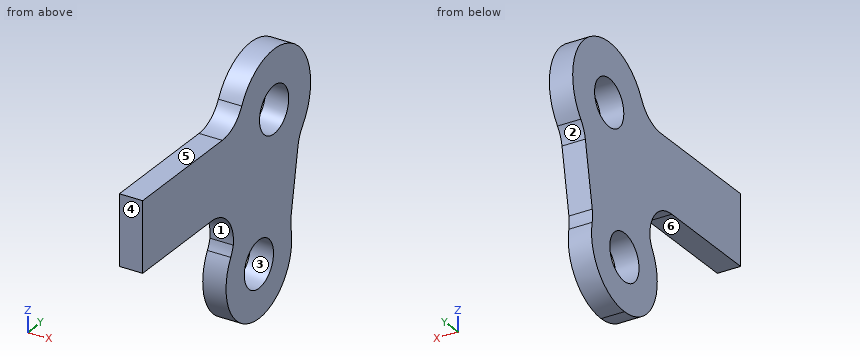
```python
from build123d import *

# Parameters (mm, degrees)
EXTRUDE_1_DEPTH          = 2
CUT_EXTRUDE_3_DEPTH      = 25.377594344
CUT_EXTRUDE_3_DEPTH_BACK = 25.377594344
SKETCH_1_3_R             = 2
FILLET_1_R               = 3


with BuildPart() as part:
    # 草图1 → 凸台-拉伸1 (new body)
    with BuildSketch(Plane(origin=(0, 0, 0), x_dir=(0, 0, -1), z_dir=(1, 0, 0))):
        with BuildLine():
            Line((0.694592711, 3.939231012), (-0.694592711, -3.939231012))
            Line((-0.694592711, -3.939231012), (3.079360166, -3.939231012))
            ThreePointArc((3.079360166, -3.939231012), (4.494263056, -2.191255253), (5, 0))
            ThreePointArc((5, 0), (4.650004293, 1.837786733), (3.64901597, 3.418286479))
            Line((3.64901597, 3.418286479), (0.694592711, 3.939231012))
        make_face()
        with BuildLine():
            Line((2.259830548, -4.460175545), (-0.694592711, -3.939231012))
            Line((-0.694592711, -3.939231012), (-0.694592711, -4.951519056))
            ThreePointArc((-0.694592711, -4.951519056), (0.820272506, -4.932256382), (2.259830548, -4.460175545))
        make_face()
        with BuildLine():
            Line((3.079360166, -3.939231012), (-0.694592711, -3.939231012))
            Line((-0.694592711, -3.939231012), (2.259830548, -4.460175545))
            ThreePointArc((2.259830548, -4.460175545), (2.68227239, -4.219646292), (3.079360166, -3.939231012))
        make_face()
        with BuildLine():
            Line((-0.694592711, -4.951519056), (-0.694592711, -3.939231012))
            Line((-0.694592711, -3.939231012), (0.694592711, 3.939231012))
            Line((0.694592711, 3.939231012), (3.64901597, 3.418286479))
            ThreePointArc((3.64901597, 3.418286479), (-4.437968609, 2.303135825), (-0.694592711, -4.951519056))
        make_face()
        with BuildLine():
            ThreePointArc((5, 0), (4.494263056, -2.191255253), (3.079360166, -3.939231012))
            Line((3.079360166, -3.939231012), (5.305407289, -3.939231012))
            Line((5.305407289, -3.939231012), (5.305407289, -4.997192896))
            Line((5.305407289, -4.997192896), (9.092867132, -5.665024255))
            ThreePointArc((9.092867132, -5.665024255), (7.386058148, -1.302361333), (10.482052554, 2.213437769))
            Line((10.482052554, 2.213437769), (3.64901597, 3.418286479))
            ThreePointArc((3.64901597, 3.418286479), (4.650004293, 1.837786733), (5, 0))
        make_face()
        with BuildLine():
            Line((5.305407289, -3.939231012), (3.079360166, -3.939231012))
            ThreePointArc((3.079360166, -3.939231012), (2.68227239, -4.219646292), (2.259830548, -4.460175545))
            Line((2.259830548, -4.460175545), (5.305407289, -4.997192896))
            Line((5.305407289, -4.997192896), (5.305407289, -3.939231012))
        make_face()
        with BuildLine():
            ThreePointArc((2.259830548, -4.460175545), (0.820272506, -4.932256382), (-0.694592711, -4.951519056))
            Line((-0.694592711, -4.951519056), (-0.694592711, -18))
            Line((-0.694592711, -18), (5.305407289, -18))
            Line((5.305407289, -18), (5.305407289, -4.997192896))
            Line((5.305407289, -4.997192896), (2.259830548, -4.460175545))
        make_face()
        with BuildLine():
            ThreePointArc((16.317693036, -2.083778132), (14.485990042, 1.539782422), (10.482052554, 2.213437769))
            Line((10.482052554, 2.213437769), (12.512285747, 1.85545288))
            Line((12.512285747, 1.85545288), (11.123100325, -6.023009144))
            Line((11.123100325, -6.023009144), (9.092867132, -5.665024255))
            ThreePointArc((9.092867132, -5.665024255), (13.816227929, -6.115633571), (16.317693036, -2.083778132))
        make_face()
        with BuildLine():
            Line((12.512285747, 1.85545288), (10.482052554, 2.213437769))
            ThreePointArc((10.482052554, 2.213437769), (7.386058148, -1.302361333), (9.092867132, -5.665024255))
            Line((9.092867132, -5.665024255), (11.123100325, -6.023009144))
            Line((11.123100325, -6.023009144), (12.512285747, 1.85545288))
        make_face()
    extrude(amount=EXTRUDE_1_DEPTH)

    # 草图1<3> → 切除-拉伸3 (cut, two sides: drawn at the far end of the back side and taken through both)
    with BuildSketch(Plane(origin=(0, 0, 0), x_dir=(0, 0, -1), z_dir=(1, 0, 0)).offset(-CUT_EXTRUDE_3_DEPTH_BACK)):
        Circle(SKETCH_1_3_R)
        with Locations((11.817693036, -2.083778132)):
            Circle(SKETCH_1_3_R)
    extrude(amount=CUT_EXTRUDE_3_DEPTH + CUT_EXTRUDE_3_DEPTH_BACK, mode=Mode.SUBTRACT)

    # 圆角1
    # the kernel refuses this fillet: 3 mm, written as the material it adds along each edge
    with BuildSketch(Plane(origin=(0, -4.951519056, 0.694592711), x_dir=(0, -1, 0), z_dir=(1, 0, 0))) as fillet_1_piece_1:
        with BuildLine():
            CenterArc((2.144253255, -3), FILLET_1_R, 90, 62.495124604)
            ThreePointArc((-0.516661362, -1.614527733), (-0.189409011, -0.829319334), (0, 0))
            Line((0, 0), (2.144253255, 0))
        make_face()
    extrude(amount=2)
    with BuildSketch(Plane(origin=(0, 3.418286479, -3.64901597), x_dir=(0, -0.17364817766699442, -0.9848077530121968), z_dir=(1, 0, 0))) as fillet_1_piece_2:
        with BuildLine():
            CenterArc((0.872983346, 3), FILLET_1_R, 241.044975628, 28.955024372)
            ThreePointArc((-0.579385409, 0.375), (-0.283214788, 0.19750856), (0, 0))
            Line((0, 0), (0.872983346, 0))
        make_face()
    extrude(amount=2)
    with BuildSketch(Plane(origin=(0, -4.997192896, -5.305407289), x_dir=(0, -0.17364817766692767, -0.9848077530122085), z_dir=(1, 0, 0))) as fillet_1_piece_3:
        with BuildLine():
            CenterArc((FILLET_1_R * 1.19175359259, -FILLET_1_R), FILLET_1_R, 90, 100)
            Line((FILLET_1_R * 0.206945839582, -FILLET_1_R * 1.17364817767), (0, 0))
            Line((0, 0), (FILLET_1_R * 1.19175359259, 0))
        make_face()
    extrude(amount=2)
    with BuildSketch(Plane(origin=(0, -5.665024255, -9.092867132), x_dir=(0, 0.17364817766698767, 0.9848077530121979), z_dir=(1, 0, 0))) as fillet_1_piece_4:
        with BuildLine():
            CenterArc((0.631029591, 3), FILLET_1_R, 248.960530219, 21.039469781)
            ThreePointArc((-0.446003371, 0.2), (-0.220284161, 0.106060125), (0, 0))
            Line((0, 0), (0.631029591, 0))
        make_face()
    extrude(amount=2)
    with BuildSketch(Plane(origin=(0, 2.213437769, -10.482052554), x_dir=(0, 0.2445079523565027, -0.9696472870247357), z_dir=(1, 0, 0))) as fillet_1_piece_5:
        with BuildLine():
            CenterArc((0.651724559, 2.995572307), FILLET_1_R, 245.847242884, 21.039469781)
            Line((-0.575787876, 0.25819889), (0, 0))
            ThreePointArc((0, 0), (0.24439671, 0.00664154), (0.488793419, 0))
        make_face()
    extrude(amount=2)


solid = part.part
```
Here's how the part is built. I have some questions about the finished solid (model axes, mm). Face numbers are marked on the shaded views. A direction names the side the tool comes from. Coordinates: 2 decimals unless noted, no trailing zeros. Loops run counter-clockwise (first coordinate to the right, second up) from the corner with the lowest first, then second, coordinate; pieces in that order, holes last. Notation, with made-up numbers: M 73,33.25 L 79,33.25 A20 ccw 79,59.25 Z; hole C 84,33.5 d7. An arc over 180 degrees is marked long. One line per item, written item: value.
1. Imagine slicing it at C-C (x = 1.3). List the corners of the cut face in (y, z) for me.
Geometry says:
outline: M -18,-5.31 L -8.57,-5.31 A3 cw -5.59,-8.65 A3 cw -5.94,-9.5 A4.5 ccw long 2.33,-10.96 A3 cw 2.32,-9.86 L 3.27,-4.51 A3 cw 3.89,-3.14 A5 ccw long -4.43,2.31 A3 cw -7.1,0.69 L -18,0.69 Z; hole C -2.08,-11.82 d4; hole C 0,0 d4
2. Will this pin go through, and if not, where does the flat tip stop? pin 1 Ø1 at (x, y) = (1, -14) entering from -Z.
Geometry says:
pin 1: stops at z = -5.31
3. Imagine slicing it at B-B (y = -3.75). List the corners of the cut face in (x, z) for me.
Geometry says:
outline: M 0,-16 L 2,-16 L 2,-12.92 L 0,-12.92 Z; M 0,-10.71 L 2,-10.71 L 2,3.31 L 0,3.31 Z
4. Thinking about a two-plate mould opening in Y: for the marked faces 1, 2 and 3, which applies, +Y half, -Y half, draft (parallel to the pull), parting line (faces both ways), or undercut?
Geometry says:
face 1: -Y half
face 2: +Y half
face 3: undercut
5. On a 3-axis mill with a long thin cutter (end or side, diameter ignored), from which of +Z, -Z, +X, -X, +Y, -Y can I reach the whole of each face in a straight line? I mean the marked faces 4, 5 and 6. Say none if no direction works.
Geometry says:
face 4: +Z, -Z, +X, -X, -Y
face 5: +Z, +X, -X, -Y
face 6: -Z, +X, -X, -Y
6. Imagine slicing it at D-D (y = -10.5). List the corners of the cut face in (x, z) for me.
Geometry says:
outline: M 0,-5.31 L 2,-5.31 L 2,0.69 L 0,0.69 Z
7. Please list where these lines run through material, in increasing order: probe 1 along Y at (x, z) = (0.7, 0); probe 2 along Z at (x, y) = (1.8, -16.5); probe 3 along Y at (x, z) = (0.6, 1.75).
Geometry says:
probe 1: y = -18 to -2, 2 to 5
probe 2: z = -5.31 to 0.69
probe 3: y = -4.81 to -0.97, 0.97 to 4.68
8. Imagine slicing it at A-A (z = 0). List the corners of the cut face in (x, y) for me, and give its area (3 significant figures).
Geometry says:
outline: M 0,-18 L 2,-18 L 2,-2 L 0,-2 Z; M 0,2 L 2,2 L 2,5 L 0,5 Z
area: 38.0 mm2
